Read the model definition and answer for the solid it produces. Units are mm, in the model's axes. A direction names the side the tool comes from. Give positions to 0.01 mm unless a question says otherwise; leave off trailing zeros. Write each loop counter-clockwise with the first axis right and the second up, starting at its lowest first coordinate (ties: lowest second). Pieces come first, ordered by that corner, then holes. Notation, with made-up numbers: (-21, 13.5) -> (33, 13.5) arc R14 cw to (33, 17.5) -> close; hole circle Ø1 at (-39, 33). An arc over 180 degrees is marked (long way). Use a Markdown table: item, result.
from build123d import *

# Parameters (mm, degrees)
SKETCH1_W             = 245.11
SKETCH1_H             = 93.653112922
BOSS_EXTRUDE1_DEPTH   = 4.318
CUT_EXTRUDE1_REACH    = 6.318
SKETCH2_W             = 4.064
SKETCH2_H             = 22.751037641
SKETCH2_W_2           = 73.236666667
SKETCH2_H_2           = 4.064
CHAMFER1_SIZE         = 0.762
CHAMFER1_SIZE2        = 1.319822715
CHAMFER1_PART_2_SIZE  = 0.762
CHAMFER1_PART_2_SIZE2 = 1.319822715
CHAMFER1_PART_3_SIZE  = 0.762
CHAMFER1_PART_3_SIZE2 = 1.319822715
CHAMFER1_PART_4_SIZE  = 0.762
CHAMFER1_PART_4_SIZE2 = 1.319822715
CHAMFER1_PART_5_SIZE  = 0.762
CHAMFER1_PART_5_SIZE2 = 1.319822715
CHAMFER1_PART_6_SIZE  = 0.762
CHAMFER1_PART_6_SIZE2 = 1.319822715
CHAMFER1_PART_7_SIZE  = 0.762
CHAMFER1_PART_7_SIZE2 = 1.319822715
CHAMFER1_PART_8_SIZE  = 0.762
CHAMFER1_PART_8_SIZE2 = 1.319822715
CHAMFER2_SIZE         = 0.762
CHAMFER2_SIZE2        = 1.319822715
CHAMFER2_PART_2_SIZE  = 0.762
CHAMFER2_PART_2_SIZE2 = 1.319822715
CHAMFER2_PART_3_SIZE  = 0.762
CHAMFER2_PART_3_SIZE2 = 1.319822715
CHAMFER2_PART_4_SIZE  = 0.762
CHAMFER2_PART_4_SIZE2 = 1.319822715
CHAMFER2_PART_5_SIZE  = 0.762
CHAMFER2_PART_5_SIZE2 = 1.319822715
CHAMFER2_PART_6_SIZE  = 0.762
CHAMFER2_PART_6_SIZE2 = 1.319822715
CHAMFER2_PART_7_SIZE  = 0.762
CHAMFER2_PART_7_SIZE2 = 1.319822715
CHAMFER2_PART_8_SIZE  = 0.762
CHAMFER2_PART_8_SIZE2 = 1.319822715


with BuildPart() as part:
    # Sketch1 → Boss-Extrude1 (new body)
    with BuildSketch(Plane(origin=(0, 0, 0), x_dir=(1, 0, 0), z_dir=(0, 1, 0))):
        Rectangle(SKETCH1_W, SKETCH1_H)
    extrude(amount=BOSS_EXTRUDE1_DEPTH)

    # Sketch2 → Cut-Extrude1 (cut, up to next)
    with BuildSketch(Plane(origin=(0, 4.318, 0), x_dir=(1, 0, 0), z_dir=(0, 1, 0)), mode=Mode.PRIVATE) as cut_extrude1_sk1:
        with Locations((-120.523, 22.751037641)):
            Rectangle(SKETCH2_W, SKETCH2_H)
    cut_extrude1_tool1 = extrude(cut_extrude1_sk1.sketch, amount=-CUT_EXTRUDE1_REACH, mode=Mode.PRIVATE) & part.part
    add(cut_extrude1_tool1.solids().sort_by_distance((-120.523, 4.318, -22.751038))[0], mode=Mode.SUBTRACT)
    # Sketch2 → Cut-Extrude1 (cut, up to next)
    with BuildSketch(Plane(origin=(0, 4.318, 0), x_dir=(1, 0, 0), z_dir=(0, 1, 0)), mode=Mode.PRIVATE) as cut_extrude1_sk2:
        with Locations((-73.236666666, -44.794556461)):
            Rectangle(SKETCH2_W_2, SKETCH2_H_2)
    cut_extrude1_tool2 = extrude(cut_extrude1_sk2.sketch, amount=-CUT_EXTRUDE1_REACH, mode=Mode.PRIVATE) & part.part
    add(cut_extrude1_tool2.solids().sort_by_distance((-73.236667, 4.318, 44.794556))[0], mode=Mode.SUBTRACT)
    # Sketch2 → Cut-Extrude1 (cut, up to next)
    with BuildSketch(Plane(origin=(0, 4.318, 0), x_dir=(1, 0, 0), z_dir=(0, 1, 0)), mode=Mode.PRIVATE) as cut_extrude1_sk3:
        with Locations((73.236666666, -44.794556461)):
            Rectangle(SKETCH2_W_2, SKETCH2_H_2)
    cut_extrude1_tool3 = extrude(cut_extrude1_sk3.sketch, amount=-CUT_EXTRUDE1_REACH, mode=Mode.PRIVATE) & part.part
    add(cut_extrude1_tool3.solids().sort_by_distance((73.236667, 4.318, 44.794556))[0], mode=Mode.SUBTRACT)
    # Sketch2 → Cut-Extrude1 (cut, up to next)
    with BuildSketch(Plane(origin=(0, 4.318, 0), x_dir=(1, 0, 0), z_dir=(0, 1, 0)), mode=Mode.PRIVATE) as cut_extrude1_sk4:
        with Locations((-120.523, -22.751037641)):
            Rectangle(SKETCH2_W, SKETCH2_H)
    cut_extrude1_tool4 = extrude(cut_extrude1_sk4.sketch, amount=-CUT_EXTRUDE1_REACH, mode=Mode.PRIVATE) & part.part
    add(cut_extrude1_tool4.solids().sort_by_distance((-120.523, 4.318, 22.751038))[0], mode=Mode.SUBTRACT)
    # Sketch2 → Cut-Extrude1 (cut, up to next)
    with BuildSketch(Plane(origin=(0, 4.318, 0), x_dir=(1, 0, 0), z_dir=(0, 1, 0)), mode=Mode.PRIVATE) as cut_extrude1_sk5:
        with Locations((-73.236666666, 44.794556461)):
            Rectangle(SKETCH2_W_2, SKETCH2_H_2)
    cut_extrude1_tool5 = extrude(cut_extrude1_sk5.sketch, amount=-CUT_EXTRUDE1_REACH, mode=Mode.PRIVATE) & part.part
    add(cut_extrude1_tool5.solids().sort_by_distance((-73.236667, 4.318, -44.794556))[0], mode=Mode.SUBTRACT)
    # Sketch2 → Cut-Extrude1 (cut, up to next)
    with BuildSketch(Plane(origin=(0, 4.318, 0), x_dir=(1, 0, 0), z_dir=(0, 1, 0)), mode=Mode.PRIVATE) as cut_extrude1_sk6:
        with Locations((73.236666666, 44.794556461)):
            Rectangle(SKETCH2_W_2, SKETCH2_H_2)
    cut_extrude1_tool6 = extrude(cut_extrude1_sk6.sketch, amount=-CUT_EXTRUDE1_REACH, mode=Mode.PRIVATE) & part.part
    add(cut_extrude1_tool6.solids().sort_by_distance((73.236667, 4.318, -44.794556))[0], mode=Mode.SUBTRACT)
    # Sketch2 → Cut-Extrude1 (cut, up to next)
    with BuildSketch(Plane(origin=(0, 4.318, 0), x_dir=(1, 0, 0), z_dir=(0, 1, 0)), mode=Mode.PRIVATE) as cut_extrude1_sk7:
        with Locations((120.523, 22.751037641)):
            Rectangle(SKETCH2_W, SKETCH2_H)
    cut_extrude1_tool7 = extrude(cut_extrude1_sk7.sketch, amount=-CUT_EXTRUDE1_REACH, mode=Mode.PRIVATE) & part.part
    add(cut_extrude1_tool7.solids().sort_by_distance((120.523, 4.318, -22.751038))[0], mode=Mode.SUBTRACT)
    # Sketch2 → Cut-Extrude1 (cut, up to next)
    with BuildSketch(Plane(origin=(0, 4.318, 0), x_dir=(1, 0, 0), z_dir=(0, 1, 0)), mode=Mode.PRIVATE) as cut_extrude1_sk8:
        with Locations((120.523, -22.751037641)):
            Rectangle(SKETCH2_W, SKETCH2_H)
    cut_extrude1_tool8 = extrude(cut_extrude1_sk8.sketch, amount=-CUT_EXTRUDE1_REACH, mode=Mode.PRIVATE) & part.part
    add(cut_extrude1_tool8.solids().sort_by_distance((120.523, 4.318, 22.751038))[0], mode=Mode.SUBTRACT)

    # Chamfer1
    chamfer1_edges = [part.edges().sort_by_distance(p)[0] for p in [
        (109.855, 2.159, -46.826556461),
    ]]
    chamfer1_side = [part.faces().sort_by_distance(p)[0] for p in [
        (116.205, 2.159, -46.826556461),
    ]]
    chamfer(chamfer1_edges, length=CHAMFER1_SIZE, length2=CHAMFER1_SIZE2, reference=chamfer1_side[0])

    # Chamfer1 part 2
    chamfer1_part_2_edges = [part.edges().sort_by_distance(p)[0] for p in [
        (-109.855, 2.159, 46.826556461),
    ]]
    chamfer1_part_2_side = [part.faces().sort_by_distance(p)[0] for p in [
        (-116.205, 2.159, 46.826556461),
    ]]
    chamfer(chamfer1_part_2_edges, length=CHAMFER1_PART_2_SIZE, length2=CHAMFER1_PART_2_SIZE2, reference=chamfer1_part_2_side[0])

    # Chamfer1 part 3
    chamfer1_part_3_edges = [part.edges().sort_by_distance(p)[0] for p in [
        (-36.618333333, 2.159, -46.826556461),
    ]]
    chamfer1_part_3_side = [part.faces().sort_by_distance(p)[0] for p in [
        (0, 2.159, -46.826556461),
    ]]
    chamfer(chamfer1_part_3_edges, length=CHAMFER1_PART_3_SIZE, length2=CHAMFER1_PART_3_SIZE2, reference=chamfer1_part_3_side[0])

    # Chamfer1 part 4
    chamfer1_part_4_edges = [part.edges().sort_by_distance(p)[0] for p in [
        (-122.555, 2.159, 11.37551882),
    ]]
    chamfer1_part_4_side = [part.faces().sort_by_distance(p)[0] for p in [
        (-122.555, 2.159, 0),
    ]]
    chamfer(chamfer1_part_4_edges, length=CHAMFER1_PART_4_SIZE, length2=CHAMFER1_PART_4_SIZE2, reference=chamfer1_part_4_side[0])

    # Chamfer1 part 5
    chamfer1_part_5_edges = [part.edges().sort_by_distance(p)[0] for p in [
        (122.555, 2.159, 34.126556461),
    ]]
    chamfer1_part_5_side = [part.faces().sort_by_distance(p)[0] for p in [
        (122.555, 2.159, 40.476556461),
    ]]
    chamfer(chamfer1_part_5_edges, length=CHAMFER1_PART_5_SIZE, length2=CHAMFER1_PART_5_SIZE2, reference=chamfer1_part_5_side[0])

    # Chamfer1 part 6
    chamfer1_part_6_edges = [part.edges().sort_by_distance(p)[0] for p in [
        (122.555, 2.159, -11.37551882),
    ]]
    chamfer1_part_6_side = [part.faces().sort_by_distance(p)[0] for p in [
        (122.555, 2.159, 0),
    ]]
    chamfer(chamfer1_part_6_edges, length=CHAMFER1_PART_6_SIZE, length2=CHAMFER1_PART_6_SIZE2, reference=chamfer1_part_6_side[0])

    # Chamfer1 part 7
    chamfer1_part_7_edges = [part.edges().sort_by_distance(p)[0] for p in [
        (36.618333333, 2.159, 46.826556461),
    ]]
    chamfer1_part_7_side = [part.faces().sort_by_distance(p)[0] for p in [
        (0, 2.159, 46.826556461),
    ]]
    chamfer(chamfer1_part_7_edges, length=CHAMFER1_PART_7_SIZE, length2=CHAMFER1_PART_7_SIZE2, reference=chamfer1_part_7_side[0])

    # Chamfer1 part 8
    chamfer1_part_8_edges = [part.edges().sort_by_distance(p)[0] for p in [
        (-122.555, 2.159, -34.126556461),
    ]]
    chamfer1_part_8_side = [part.faces().sort_by_distance(p)[0] for p in [
        (-122.555, 2.159, -40.476556461),
    ]]
    chamfer(chamfer1_part_8_edges, length=CHAMFER1_PART_8_SIZE, length2=CHAMFER1_PART_8_SIZE2, reference=chamfer1_part_8_side[0])

    # Chamfer2
    chamfer2_edges = [part.edges().sort_by_distance(p)[0] for p in [
        (36.618333333, 2.159, -46.826556461),
    ]]
    chamfer2_side = [part.faces().sort_by_distance(p)[0] for p in [
        (0.381, 2.159, -46.826556461),
    ]]
    chamfer(chamfer2_edges, length=CHAMFER2_SIZE, length2=CHAMFER2_SIZE2, reference=chamfer2_side[0])

    # Chamfer2 part 2
    chamfer2_part_2_edges = [part.edges().sort_by_distance(p)[0] for p in [
        (-36.618333333, 2.159, 46.826556461),
    ]]
    chamfer2_part_2_side = [part.faces().sort_by_distance(p)[0] for p in [
        (-0.381, 2.159, 46.826556461),
    ]]
    chamfer(chamfer2_part_2_edges, length=CHAMFER2_PART_2_SIZE, length2=CHAMFER2_PART_2_SIZE2, reference=chamfer2_part_2_side[0])

    # Chamfer2 part 3
    chamfer2_part_3_edges = [part.edges().sort_by_distance(p)[0] for p in [
        (-109.855, 2.159, -46.826556461),
    ]]
    chamfer2_part_3_side = [part.faces().sort_by_distance(p)[0] for p in [
        (-116.205, 2.159, -46.826556461),
    ]]
    chamfer(chamfer2_part_3_edges, length=CHAMFER2_PART_3_SIZE, length2=CHAMFER2_PART_3_SIZE2, reference=chamfer2_part_3_side[0])

    # Chamfer2 part 4
    chamfer2_part_4_edges = [part.edges().sort_by_distance(p)[0] for p in [
        (-122.555, 2.159, 34.126556461),
    ]]
    chamfer2_part_4_side = [part.faces().sort_by_distance(p)[0] for p in [
        (-122.555, 2.159, 40.476556461),
    ]]
    chamfer(chamfer2_part_4_edges, length=CHAMFER2_PART_4_SIZE, length2=CHAMFER2_PART_4_SIZE2, reference=chamfer2_part_4_side[0])

    # Chamfer2 part 5
    chamfer2_part_5_edges = [part.edges().sort_by_distance(p)[0] for p in [
        (122.555, 2.159, 11.37551882),
    ]]
    chamfer2_part_5_side = [part.faces().sort_by_distance(p)[0] for p in [
        (122.555, 2.159, 0.381),
    ]]
    chamfer(chamfer2_part_5_edges, length=CHAMFER2_PART_5_SIZE, length2=CHAMFER2_PART_5_SIZE2, reference=chamfer2_part_5_side[0])

    # Chamfer2 part 6
    chamfer2_part_6_edges = [part.edges().sort_by_distance(p)[0] for p in [
        (122.555, 2.159, -34.126556461),
    ]]
    chamfer2_part_6_side = [part.faces().sort_by_distance(p)[0] for p in [
        (122.555, 2.159, -40.476556461),
    ]]
    chamfer(chamfer2_part_6_edges, length=CHAMFER2_PART_6_SIZE, length2=CHAMFER2_PART_6_SIZE2, reference=chamfer2_part_6_side[0])

    # Chamfer2 part 7
    chamfer2_part_7_edges = [part.edges().sort_by_distance(p)[0] for p in [
        (109.855, 2.159, 46.826556461),
    ]]
    chamfer2_part_7_side = [part.faces().sort_by_distance(p)[0] for p in [
        (116.205, 2.159, 46.826556461),
    ]]
    chamfer(chamfer2_part_7_edges, length=CHAMFER2_PART_7_SIZE, length2=CHAMFER2_PART_7_SIZE2, reference=chamfer2_part_7_side[0])

    # Chamfer2 part 8
    chamfer2_part_8_edges = [part.edges().sort_by_distance(p)[0] for p in [
        (-122.555, 2.159, -11.37551882),
    ]]
    chamfer2_part_8_side = [part.faces().sort_by_distance(p)[0] for p in [
        (-122.555, 2.159, -0.381),
    ]]
    chamfer(chamfer2_part_8_edges, length=CHAMFER2_PART_8_SIZE, length2=CHAMFER2_PART_8_SIZE2, reference=chamfer2_part_8_side[0])


solid = part.part
Item 1: A cutting plane is placed at A-A (z = 23). Give the vertices of the cut face in (x, y).
Return value:
| item | result |
|---|---|
| outline | (-118.49, 0) -> (118.49, 0) -> (118.49, 4.32) -> (-118.49, 4.32) -> close |
Item 2: Each of these flat-tipped pins is pushed along its axis until it touches: P1, Ø1.3, axis at y = 2, z = 27.5, coming from the -X side; P2, Ø2, axis at x = 57.5, y = 2.5, coming from the -Z side; P3, Ø1, axis at x = -80.5, y = 3, coming from the +Z side; P4, Ø2, axis at x = -45.5, z = -12, coming from the -Y side. Where does it stop, or does it pass through?
Return value:
| item | result |
|---|---|
| P1 | x = -118.49 |
| P2 | z = -42.76 |
| P3 | z = 42.76 |
| P4 | y = 0 |
Item 3: Straight lines are drawn through the part: line 1 along Z through (x, y) = (85.5, 3.8); line 2 along X through (y, z) = (0.45, 17.5). For each, find the intervals that lie inside material, in ascending order. Write a range as [from, to].
Return value:
| item | result |
|---|---|
| line 1 | [-42.76, 42.76] |
| line 2 | [-118.49, 118.49] |
Item 4: A tool of negligible diameter and unlimited length cuts with its end or side. For faces 4 (the face through (-74, 2, 42.763)), 5 (the face through (122.555, 2, 0)), 6 (the face through (118.491, 2, -23)), 7 (the face through (-118.491, 2, -23)), 8 (the face through (73, 2, -42.763)), from which of +Z, -Z, +X, -X, +Y, -Y can it reach the whole face along a straight path? Write none if from no direction.
Return value:
| item | result |
|---|---|
| face 4 | +Z, +Y, -Y |
| face 5 | +Z, -Z, +X, +Y, -Y |
| face 6 | +X, +Y, -Y |
| face 7 | -X, +Y, -Y |
| face 8 | -Z, +Y, -Y |
Item 5: For a pull along X with two mould halves and no side action, classify faces 1 (the face through (-2, 4.318, -1)), 2 (the face through (73, 2, 42.763)), 3 (the face through (-118.491, 2, 23)) as +X half, -X half, draft (parallel to the pull), parting line (faces both ways), or undercut.
Return value:
| item | result |
|---|---|
| face 1 | draft |
| face 2 | undercut |
| face 3 | -X half |
Item 6: A cutting plane is placed at B-B (x = -101). Give the vertices of the cut face in (y, z), then the cut area to 3 significant figures.
Return value:
| item | result |
|---|---|
| outline | (0, -42.76) -> (4.32, -42.76) -> (4.32, 42.76) -> (0, 42.76) -> close |
| area | 369 mm^2 |
